from build123d import *

# Parameters (mm, degrees)
SKETCH1_W           = 30
SKETCH1_H           = 10
SKETCH1_R           = 3.5
BOSS_EXTRUDE1_DEPTH = 1.5
SKETCH2_W           = 30
SKETCH2_H           = 10
SKETCH2_R           = 2.25
BOSS_EXTRUDE2_DEPTH = 4


with BuildPart() as part:
    # Sketch1 → Boss-Extrude1 (new body)
    with BuildSketch(Plane.XY):
        Rectangle(SKETCH1_W, SKETCH1_H)
        with Locations((-9.375, 0)):
            Circle(SKETCH1_R, mode=Mode.SUBTRACT)
        with Locations((9.375, 0)):
            Circle(SKETCH1_R, mode=Mode.SUBTRACT)
    extrude(amount=BOSS_EXTRUDE1_DEPTH)

    # Sketch2 → Boss-Extrude2 (add)
    with BuildSketch(Plane.XY.offset(1.5)):
        Rectangle(SKETCH2_W, SKETCH2_H)
        with Locations((-9.375, 0)):
            Circle(SKETCH2_R, mode=Mode.SUBTRACT)
        with Locations((9.375, 0)):
            Circle(SKETCH2_R, mode=Mode.SUBTRACT)
    extrude(amount=BOSS_EXTRUDE2_DEPTH)


solid = part.part
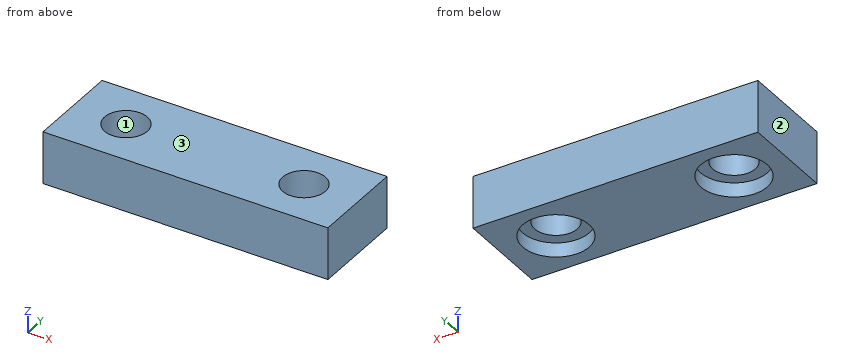
Can you work these out from the model? Positions are in its coordinate system, mm. Face numbers are marked on the shaded views. Coordinates: 2 decimals unless noted, no trailing zeros. Order: outer loops, then holes, each group sorted by start corner. A loop starts at its lowest first (then second) coordinate and runs counter-clockwise, first axis right, second up. Notation, with made-up numbers: (64, 44) -> (104, 44) arc R15 cw to (104, 73) -> close; hole circle Ø3 at (-0.75, 34.25). An arc over 180 degrees is marked (long way). Use one line per item in the form item = value.
Q1. We'd pull the mould along X, two halves only. Please class the marked faces 1, 2 and 3: released by +X, released by -X, zero draft, split by the parting line, or undercut.
From the geometry:
face_1 = undercut
face_2 = released by -X
face_3 = zero draft
Q2. Imagine slicing it at C-C, the plane y = 2.75. List the corners of the cut face in (x, z) for me.
From the geometry:
outline = (-15, 0) -> (-11.54, 0) -> (-11.54, 1.5) -> (-7.21, 1.5) -> (-7.21, 0) -> (7.21, 0) -> (7.21, 1.5) -> (11.54, 1.5) -> (11.54, 0) -> (15, 0) -> (15, 5.5) -> (-15, 5.5) -> close
Q3. Imagine slicing it at B-B, the plane z = 1. List the corners of the cut face in (x, y) for me (3 decimals), then the cut area to 3 significant figures.
From the geometry:
outline = (-15, -5) -> (15, -5) -> (15, 5) -> (-15, 5) -> close; hole circle Ø7 at (-9.375, 0); hole circle Ø7 at (9.375, 0)
area = 223 mm²
Q4. Will this pin go through, and if not, where does the flat tip stop? P1, Ø5.5, axis at x = -10, y = 0, coming from the -Z side.
From the geometry:
P1 = 1.5
Q5. I need wall thicknesses on L1, parallel to X at y = -0.75, z = 1.3; L2, parallel to X at y = -2, z = 2.2; L3, parallel to Z at x = -9.75, y = 2.5. Which ranges of each line are inside material? Lowest first, please.
From the geometry:
L1 = -15 to -12.79, -5.96 to 5.96, 12.79 to 15
L2 = -15 to -10.41, -8.34 to 8.34, 10.41 to 15
L3 = 1.5 to 5.5
Q6. Imagine slicing it at A-A, the plane y = 0. List the corners of the cut face in (x, z) for me (3 decimals).
From the geometry:
outline = (-15, 0) -> (-12.875, 0) -> (-12.875, 1.5) -> (-11.625, 1.5) -> (-11.625, 5.5) -> (-15, 5.5) -> close; (-7.125, 1.5) -> (-5.875, 1.5) -> (-5.875, 0) -> (5.875, 0) -> (5.875, 1.5) -> (7.125, 1.5) -> (7.125, 5.5) -> (-7.125, 5.5) -> close; (11.625, 1.5) -> (12.875, 1.5) -> (12.875, 0) -> (15, 0) -> (15, 5.5) -> (11.625, 5.5) -> close
